Here's how the part is built. I have some questions about the finished solid (model axes, mm). Face numbers are marked on the shaded views. A direction names the side the tool comes from. Round coordinates to 2 decimals unless told otherwise and drop trailing zeros. Loops run counter-clockwise (first coordinate to the right, second up) from the corner with the lowest first, then second, coordinate; pieces in that order, holes last. Notation, with made-up numbers: (61.25, -15.5) -> (92.25, -15.5) arc R23 ccw to (92.25, 1.5) -> close; hole circle Ø9 at (-32.5, 5.5). An arc over 180 degrees is marked (long way). Use CSV: the item, a comma, the result in double quotes. Start each with the question number.
from build123d import *

# Parameters (mm, degrees)
BOSS_EXTRUDE1_DEPTH = 5


with BuildPart() as part:
    # Sketch1 → Boss-Extrude1 (new, symmetric)
    with BuildSketch(Plane.XY):
        with BuildLine():
            ThreePointArc((-9.841451141, 11.320151918), (-10.606601718, 10.606601718), (-11.320151918, 9.841451141))
            ThreePointArc((-11.320151918, 9.841451141), (-13.628216731, 9.32005242), (-14.818281553, 11.36523347))
            ThreePointArc((-14.818281553, 11.36523347), (-18.926875967, 17.70515779), (-25.980762114, 15))
            ThreePointArc((-25.980762114, 15), (-30, 0), (-25.980762114, -15))
            ThreePointArc((-25.980762114, -15), (-18.926875967, -17.70515779), (-14.818281553, -11.36523347))
            ThreePointArc((-14.818281553, -11.36523347), (-13.628216731, -9.32005242), (-11.320151918, -9.841451141))
            ThreePointArc((-11.320151918, -9.841451141), (-10.606601718, -10.606601718), (-9.841451141, -11.320151918))
            ThreePointArc((-9.841451141, -11.320151918), (-9.32005242, -13.628216731), (-11.36523347, -14.818281553))
            ThreePointArc((-11.36523347, -14.818281553), (-17.70515779, -18.926875967), (-15, -25.980762114))
            ThreePointArc((-15, -25.980762114), (0, -30), (15, -25.980762114))
            ThreePointArc((15, -25.980762114), (17.70515779, -18.926875967), (11.36523347, -14.818281553))
            ThreePointArc((11.36523347, -14.818281553), (9.32005242, -13.628216731), (9.841451141, -11.320151918))
            ThreePointArc((9.841451141, -11.320151918), (10.606601718, -10.606601718), (11.320151918, -9.841451141))
            ThreePointArc((11.320151918, -9.841451141), (13.628216731, -9.32005242), (14.818281553, -11.36523347))
            ThreePointArc((14.818281553, -11.36523347), (18.926875967, -17.70515779), (25.980762114, -15))
            ThreePointArc((25.980762114, -15), (30, 0), (25.980762114, 15))
            ThreePointArc((25.980762114, 15), (18.926875967, 17.70515779), (14.818281553, 11.36523347))
            ThreePointArc((14.818281553, 11.36523347), (13.628216731, 9.32005242), (11.320151918, 9.841451141))
            ThreePointArc((11.320151918, 9.841451141), (10.606601718, 10.606601718), (9.841451141, 11.320151918))
            ThreePointArc((9.841451141, 11.320151918), (9.32005242, 13.628216731), (11.36523347, 14.818281553))
            ThreePointArc((11.36523347, 14.818281553), (17.70515779, 18.926875967), (15, 25.980762114))
            ThreePointArc((15, 25.980762114), (0, 30), (-15, 25.980762114))
            ThreePointArc((-15, 25.980762114), (-17.70515779, 18.926875967), (-11.36523347, 14.818281553))
            ThreePointArc((-11.36523347, 14.818281553), (-9.32005242, 13.628216731), (-9.841451141, 11.320151918))
        make_face()
        with BuildLine():
            ThreePointArc((13.5, 23.382685902), (0, 27), (-13.5, 23.382685902))
            ThreePointArc((-13.5, 23.382685902), (-14.598076211, 19.284609691), (-10.5, 18.186533479))
            ThreePointArc((-10.5, 18.186533479), (0, 21), (10.5, 18.186533479))
            ThreePointArc((10.5, 18.186533479), (14.598076211, 19.284609691), (13.5, 23.382685902))
        make_face(mode=Mode.SUBTRACT)
        with BuildLine():
            ThreePointArc((23.382685902, -13.5), (27, 0), (23.382685902, 13.5))
            ThreePointArc((23.382685902, 13.5), (19.284609691, 14.598076211), (18.186533479, 10.5))
            ThreePointArc((18.186533479, 10.5), (21, 0), (18.186533479, -10.5))
            ThreePointArc((18.186533479, -10.5), (19.284609691, -14.598076211), (23.382685902, -13.5))
        make_face(mode=Mode.SUBTRACT)
        with BuildLine():
            ThreePointArc((-13.5, -23.382685902), (0, -27), (13.5, -23.382685902))
            ThreePointArc((13.5, -23.382685902), (14.598076211, -19.284609691), (10.5, -18.186533479))
            ThreePointArc((10.5, -18.186533479), (0, -21), (-10.5, -18.186533479))
            ThreePointArc((-10.5, -18.186533479), (-14.598076211, -19.284609691), (-13.5, -23.382685902))
        make_face(mode=Mode.SUBTRACT)
        with BuildLine():
            ThreePointArc((-23.382685902, 13.5), (-27, 0), (-23.382685902, -13.5))
            ThreePointArc((-23.382685902, -13.5), (-19.284609691, -14.598076211), (-18.186533479, -10.5))
            ThreePointArc((-18.186533479, -10.5), (-21, 0), (-18.186533479, 10.5))
            ThreePointArc((-18.186533479, 10.5), (-19.284609691, 14.598076211), (-23.382685902, 13.5))
        make_face(mode=Mode.SUBTRACT)
    extrude(amount=BOSS_EXTRUDE1_DEPTH, both=True)


solid = part.part
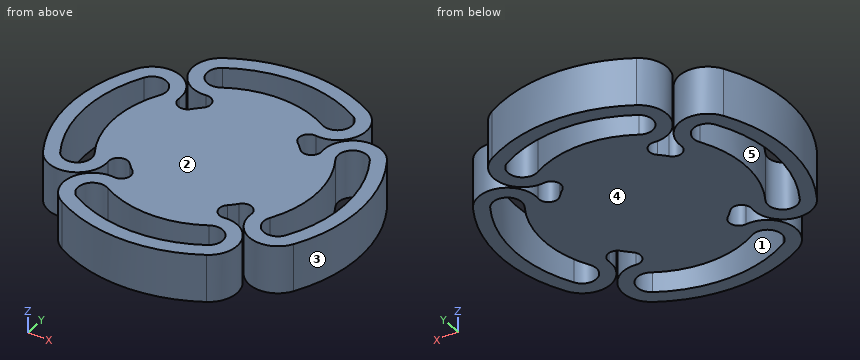
Q1. I want a section at B-B, the plane y = -24.5. List the corners of the cut face in (x, z) for me, then the cut area to 3 significant figures.
Q2. Will this pin go through, and if not, where does the flat tip stop? pin 1 Ø2 at (y, z) = (-14.5, 1) entering from -X.
Q3. For the marked faces 4 and 5, which set-ups out of +Z, -Z, +X, -X, +Y, -Y let a thin tool reach every point of the face, with its end or its side?
Q4. If we mould it in two halves opening along Y, with no side actions, what happens to the marked faces 1, 2 and 3? For each: pulls with the +Y half, pulls with the -Y half, needs draft (parallel to the pull), parting line crosses it, or undercut.
Q5. I want a section at A-A, the plane y = -7. List the corners of the cut face in (x, z) for me, then the cut area to 3 significant figures.
Q6. I want a section at D-D, the plane y = 4.5. List the corners of the cut face in (x, z) for me, then the cut area to 3 significant figures.
Q7. I want a section at C-C, the plane z = 3. Count the separate pieces of the cut face and the enclosed holes in it, then the cut area to 3 significant figures.
Q8. I need wall thicknesses on line 1 along Y through (x, z) = (13, -4); line 2 along Y through (x, z) = (-4, 1.25); line 3 along X through (y, z) = (2.5, 2). Which ranges of each line are inside material? Lowest first, please.
Values found:
1,outline,"(-16.71, -5) -> (-11.35, -5) -> (-11.35, 5) -> (-16.71, 5) -> close; (11.35, -5) -> (16.71, -5) -> (16.71, 5) -> (11.35, 5) -> close"
1,area,"107 mm2"
2,pin 1,"x = -26.79"
3,face 4,"-Z, +X, -X, +Y, -Y"
3,face 5,"+Z, -Z"
4,face 1,"undercut"
4,face 2,"needs draft"
4,face 3,"parting line crosses it"
5,outline,"(-29.17, -5) -> (-26.08, -5) -> (-26.08, 5) -> (-29.17, 5) -> close; (-19.8, -5) -> (19.8, -5) -> (19.8, 5) -> (-19.8, 5) -> close; (26.08, -5) -> (29.17, -5) -> (29.17, 5) -> (26.08, 5) -> close"
5,area,"458 mm2"
6,outline,"(-29.66, -5) -> (-26.62, -5) -> (-26.62, 5) -> (-29.66, 5) -> close; (-20.51, -5) -> (20.51, -5) -> (20.51, 5) -> (-20.51, 5) -> close; (26.62, -5) -> (29.66, -5) -> (29.66, 5) -> (26.62, 5) -> close"
6,area,"471 mm2"
7,separate pieces,"1"
7,enclosed holes,"4"
7,area,"1,890 mm2"
8,line 1,"-27.04 to -23.66, -17.96 to -14.87, -9.16 to 9.16, 14.87 to 17.96, 23.66 to 27.04"
8,line 2,"-29.73 to -26.7, -20.62 to 20.62, 26.7 to 29.73"
8,line 3,"-29.9 to -26.88, -20.85 to 20.85, 26.88 to 29.9"
